Part model, mm, in its own coordinate system. A direction names the side the tool comes from. Give positions to 0.01 mm unless a question says otherwise; leave off trailing zeros. Order: outer loops, then holes, each group sorted by start corner. A loop starts at its lowest first (then second) coordinate and runs counter-clockwise, first axis right, second up. Notation, with made-up numbers: M -32,28.25 L -11,28.25 A35 cw -11,60.25 Z; hole C 1,-3.75 d5. An arc over 180 degrees is marked long. Write each question's results on one line, items separated by ' | '. Start each with the question number.
from build123d import *

# Parameters (mm, degrees)
SKETCH1_R           = 250
SKETCH1_R_2         = 180
SKETCH1_R_3         = 12.5
BOSS_EXTRUDE1_DEPTH = 20


# Read off the part's stored shape, not the designer's step: Revolve1
with BuildPart() as part:
    # Sketch1 → Boss-Extrude1 (new body)
    with BuildSketch(Plane(origin=(0, 0, 0), x_dir=(1, 0, 0), z_dir=(0, 1, 0))):
        with Locations(Location((0, 0, 0), (0, 0, 270))):
            Circle(SKETCH1_R)
        with Locations(Location((0, 0, 0), (0, 0, 270))):
            Circle(SKETCH1_R_2, mode=Mode.SUBTRACT)
        with Locations(Location((0, 217.5, 0), (0, 0, 270))):
            Circle(SKETCH1_R_3, mode=Mode.SUBTRACT)
        with Locations(Location((108.75, 188.360525323, 0), (0, 0, 270))):
            Circle(SKETCH1_R_3, mode=Mode.SUBTRACT)
        with Locations(Location((188.360525323, 108.75, 0), (0, 0, 270))):
            Circle(SKETCH1_R_3, mode=Mode.SUBTRACT)
        with Locations(Location((217.5, 0, 0), (0, 0, 270))):
            Circle(SKETCH1_R_3, mode=Mode.SUBTRACT)
        with Locations(Location((188.360525323, -108.75, 0), (0, 0, 270))):
            Circle(SKETCH1_R_3, mode=Mode.SUBTRACT)
        with Locations(Location((108.75, -188.360525323, 0), (0, 0, 270))):
            Circle(SKETCH1_R_3, mode=Mode.SUBTRACT)
        with Locations(Location((0, -217.5, 0), (0, 0, 270))):
            Circle(SKETCH1_R_3, mode=Mode.SUBTRACT)
        with Locations(Location((-108.75, -188.360525323, 0), (0, 0, 270))):
            Circle(SKETCH1_R_3, mode=Mode.SUBTRACT)
        with Locations(Location((-188.360525323, -108.75, 0), (0, 0, 270))):
            Circle(SKETCH1_R_3, mode=Mode.SUBTRACT)
        with Locations(Location((-217.5, 0, 0), (0, 0, 270))):
            Circle(SKETCH1_R_3, mode=Mode.SUBTRACT)
        with Locations(Location((-188.360525323, 108.75, 0), (0, 0, 270))):
            Circle(SKETCH1_R_3, mode=Mode.SUBTRACT)
        with Locations(Location((-108.75, 188.360525323, 0), (0, 0, 270))):
            Circle(SKETCH1_R_3, mode=Mode.SUBTRACT)
    extrude(amount=BOSS_EXTRUDE1_DEPTH)

    # Revolve1 outline → Revolve1 (revolve)
    with BuildSketch(Plane.XY):
        with BuildLine():
            ThreePointArc((205, 19.9999999), (144.956890179, 164.956890108), (0, 225))
            Line((0, 225), (0, 200))
            ThreePointArc((0, 200), (127.279220649, 147.279220578), (180, 19.9999999))
            Line((180, 19.9999999), (205, 19.9999999))
        make_face()
    revolve(axis=Axis((0, 0, 0), (0, 1, 0)))


solid = part.part
(1) Probe L1, parallel to X at y = 8, z = 0; L2, parallel to Y at x = -193, z = -147.5; L3, parallel to Z at x = 180.5, y = 18. List the from-to ranges inside material, lowest first.
(2) Saw through at A-A on x = 217.5. Give the cut face in (y, z).
(3) Pull direction Z, two halves, no side cores. Call faces 3 (the cylindrical face through (-205.106, 9.86, -1.627)), 4 (the cylindrical face through (10.99, 9.86, -249.76)), 5 (the flat face through (205, 20, 17)): +Z half, -Z half, draft (parallel to the pull), parting line (faces both ways), or undercut.
(4) Tool access for faces 1 (the cylindrical face through (-68.941, 9.86, 166.274)), 2 (the cylindrical face through (-177.82, 9.86, -102.03)): list every direction of +Z, -Z, +X, -X, +Y, -Y with a clear straight run to the whole face (end or side of a thin tool).
(5) Saw through at B-B on z = 108.75. Give the cut face in (x, y), plus the area to 3 significant figures.
(6) Drop flat-ended pins along their axis: P1, Ø3, axis at x = 139, z = -84.5, coming from the +Y side; P2, Ø1.5, axis at y = 51.5, z = 0.5, coming from the +X side; P3, Ø4, axis at y = 141.5, z = -58, coming from the -X side. Give the stop position or say it passes through.
(7) Saw through at D-D on z = -217.5. Give the cut face in (x, y).
(8) Saw through at C-C on x = 108.75. Give the cut face in (y, z), plus the area to 3 significant figures.
Taken from the geometry:
1) L1: x = -250 to -230, -205 to -180, 180 to 205, 230 to 250 | L2: y = 0 to 20 | L3: z = -172.97 to -118.47, -99.03 to 99.03, 118.47 to 172.97
2) outline: M 0,-123.26 L 20,-123.26 L 20,-12.5 L 0,-12.5 Z; M 0,12.5 L 20,12.5 L 20,123.26 L 0,123.26 Z
3) face 3: undercut | face 4: parting line | face 5: draft
4) face 1: -Y | face 2: +Y, -Y
5) outline: M -225.11,0 L -200.86,0 L -200.86,20 L -225.11,20 Z; M -175.86,0 L -143.43,0 L -143.43,20 A143.43 cw 143.43,20 L 143.43,0 L 175.86,0 L 175.86,20 L 173.78,20 A173.78 ccw -173.78,20 L -175.86,20 Z; M 200.86,0 L 225.11,0 L 225.11,20 L 200.86,20 Z | area: 17,400 mm²
6) P1: stops at y = 146.69 | P2: stops at x = 202.68 | P3: stops at x = -156.31
7) outline: M -123.26,0 L -12.5,0 L -12.5,20 L -123.26,20 Z; M 12.5,0 L 123.26,0 L 123.26,20 L 12.5,20 Z
8) outline: M 0,-225.11 L 20,-225.11 L 20,-200.86 L 0,-200.86 Z; M 0,-175.86 L 20,-175.86 L 20,-173.78 A173.78 ccw 20,173.78 L 20,175.86 L 0,175.86 L 0,143.43 L 20,143.43 A143.43 cw 20,-143.43 L 0,-143.43 Z; M 0,200.86 L 20,200.86 L 20,225.11 L 0,225.11 Z | area: 17,400 mm²
